Source: CAD feature listing. Evaluate the final solid. Frame: model axes, mm. A direction names the side the tool comes from. Coordinates: 2 decimals unless noted, no trailing zeros. Loops run counter-clockwise (first coordinate to the right, second up) from the corner with the lowest first, then second, coordinate; pieces in that order, holes last. Notation, with made-up numbers: (-4, -12) -> (13, -12) arc R16 ccw to (13, 2) -> close; hole circle Ø10 at (62, 9.25). An arc over 180 degrees is marked (long way). One line per question, with ' | ' between items. Start each with the question number.
```python
from build123d import *

# Parameters (mm, degrees)
F0_W      = 66
F0_H      = 38
F1_DEPTH  = 2
F2_W      = 66
F2_H      = 38
F2_W_2    = 62
F2_H_2    = 34
F3_DEPTH  = 10
F4_SIZE   = 1
F5_R      = 2
F6_R      = 1
F7_W      = 5.2
F7_H      = 34
F8_DEPTH  = 3
F9_R      = 1.5
F10_DEPTH = 38.001
F11_W     = 4
F11_H     = 10.8
F12_DEPTH = 7
F13_R     = 1.5
F14_DEPTH = 38.001


with BuildPart() as f1:
    # F0 (on Top) → F1 (new body)
    with BuildSketch(Plane.XY):
        with Locations((33, -19)):
            Rectangle(F0_W, F0_H)
    extrude(amount=F1_DEPTH)

    # F2 (on face) → F3 (join)
    with BuildSketch(Plane.XY.offset(2)):
        with Locations((33, -19)):
            Rectangle(F2_W, F2_H)
        with Locations((33, -19)):
            Rectangle(F2_W_2, F2_H_2, mode=Mode.SUBTRACT)
    extrude(amount=F3_DEPTH)

    # F4
    f4_edges = [f1.edges().sort_by_distance(p)[0] for p in [
        (2, -2, 7),
        (2, -36, 7),
        (64, -2, 7),
        (64, -36, 7),
    ]]
    chamfer(f4_edges, length=F4_SIZE)

    # F5
    f5_edges = [f1.edges().sort_by_distance(p)[0] for p in [
        (0, -38, 6),
        (66, -38, 6),
        (66, 0, 6),
        (0, 0, 6),
    ]]
    fillet(f5_edges, radius=F5_R)

    # F6
    f6_edges = [f1.edges().sort_by_distance(p)[0] for p in [
        (0, -19, 12),
        (33, -38, 12),
        (66, -19, 12),
        (33, 0, 12),
    ]]
    fillet(f6_edges, radius=F6_R)

    # F7 (on face) → F8 (join)
    with BuildSketch(Plane.XY.offset(2)):
        with Locations((4.6, -19)):
            Rectangle(F7_W, F7_H)
        with Locations((61.4, -19)):
            Rectangle(F7_W, F7_H)
    extrude(amount=F8_DEPTH)

    # F9 (on face) → F10 (cut, through all)
    with BuildSketch(Plane.XZ.offset(38)):
        with Locations((3.7, 2.5)):
            Circle(F9_R)
        with Locations((62.3, 2.5)):
            Circle(F9_R)
    extrude(amount=-F10_DEPTH, mode=Mode.SUBTRACT)

    # F11 (on face) → F12 (join)
    with BuildSketch(Plane.XY.offset(5)):
        with Locations((5.2, -8.6)):
            Rectangle(F11_W, F11_H)
        with Locations((5.2, -29.4)):
            Rectangle(F11_W, F11_H)
        with Locations((60.8, -8.6)):
            Rectangle(F11_W, F11_H)
        with Locations((60.8, -29.4)):
            Rectangle(F11_W, F11_H)
    extrude(amount=F12_DEPTH)

    # F13 (on face) → F14 (cut, through all)
    with BuildSketch(Plane.XZ.offset(38)):
        with Locations((5, 9)):
            Circle(F13_R)
        with Locations((61, 9)):
            Circle(F13_R)
    extrude(amount=-F14_DEPTH, mode=Mode.SUBTRACT)


solid = f1.part
```
(1) Access query for faces 4 (the flat face through (62.8, -29, 8)), 5 (the flat face through (61, -9, 12)). Directions: +Z, -Z, +X, -X, +Y, -Y. A direction counts if a zero-diameter tool reaches every point of the face in a straight line with its end or side. Return the directions, or none.
(2) Cut plane D-D, the plane z = 9. State how many separate pieces and enclosed holes the cut face has, and give its area (3 significant figures).
(3) Ray query, L1, parallel to Y at x = 55.5, z = 2.75; L2, parallel to Z at x = 61, y = -1.45; L3, parallel to X at y = -11.5, z = 11.25. Return the intervals inside material, ascending.
(4) Cut plane C-C, the plane x = 23. Return the cut outline in (y, z), and give its area (3 significant figures).
(5) Cut plane A-A, the plane y = -18. Return the cut outline in (x, z).
(6) Contact query for flat-ended pins moving along their axis: pin 1 Ø1.2 at (x, z) = (60, 10) entering from -Y; pin 2 Ø4 at (x, y) = (23.5, -28) entering from +Z; pin 3 Ø1.2 at (x, z) = (5.5, 9) entering from -Y. Output: stop coordinate, or through.
(7) Cut plane B-B, the plane y = -27. Return the cut outline in (x, z), and give its area (3 significant figures).
(8) Draft query along Z for faces 1 (the flat face through (33, 0, 5)), 2 (the flat face through (5, -9, 12)), 3 (the cylindrical face through (61.1, -19.3, 1.6)). Return one class per face: pulls with the +Z half, pulls with the -Z half, needs draft (parallel to the pull), parting line crosses it, or undercut.
Here are the results:
1) face 4: +Z | face 5: +Z, +X, -X, +Y, -Y
2) separate pieces: 12 | enclosed holes: 0 | area: 418 mm2
3) L1: y = -38 to -36, -2 to 0 | L2: z = 0 to 1.75, 3.25 to 7.5, 10.5 to 12 | L3: x = 0.03 to 2, 3.2 to 7.2, 58.8 to 62.8, 64 to 65.97
4) outline: (-38, 0) -> (0, 0) -> (0, 11) arc R1 ccw to (-1, 12) -> (-2, 12) -> (-2, 2) -> (-36, 2) -> (-36, 12) -> (-37, 12) arc R1 ccw to (-38, 11) -> close | area: 116 mm2
5) outline: (0, 0) -> (66, 0) -> (66, 11) arc R1 ccw to (65, 12) -> (64, 12) -> (64, 5) -> (58.8, 5) -> (58.8, 2) -> (7.2, 2) -> (7.2, 5) -> (2, 5) -> (2, 12) -> (1, 12) arc R1 ccw to (0, 11) -> close; hole circle Ø3 at (3.7, 2.5); hole circle Ø3 at (62.3, 2.5)
6) pin 1: stops at y = -38 | pin 2: stops at z = 2 | pin 3: passes through
7) outline: (0, 0) -> (66, 0) -> (66, 11) arc R1 ccw to (65, 12) -> (64, 12) -> (64, 5) -> (62.8, 5) -> (62.8, 12) -> (58.8, 12) -> (58.8, 2) -> (7.2, 2) -> (7.2, 12) -> (3.2, 12) -> (3.2, 5) -> (2, 5) -> (2, 12) -> (1, 12) arc R1 ccw to (0, 11) -> close; hole circle Ø3 at (3.7, 2.5); hole circle Ø3 at (5, 9); hole circle Ø3 at (61, 9); hole circle Ø3 at (62.3, 2.5) | area: 230 mm2
8) face 1: needs draft | face 2: pulls with the +Z half | face 3: undercut
